Study the drawing (mm; zero at the part's minimum x, y, z) and answer. A direction names the side the tool comes from. Give positions to 0.01 mm unless a question says otherwise; leave off trailing zeros. Loops run counter-clockwise (first coordinate to the right, second up) from the corner with the lowest first, then second, coordinate; pieces in that order, holes last. Notation, with made-up numbers: (70.25, 45.25) - (78.25, 45.25) arc R12 cw to (78.25, 61.25) - close; hole circle Ø1 at (58, -36.75). An arc over 180 degrees is marked (long way). One line per item, written item: value. Start each with the question number.
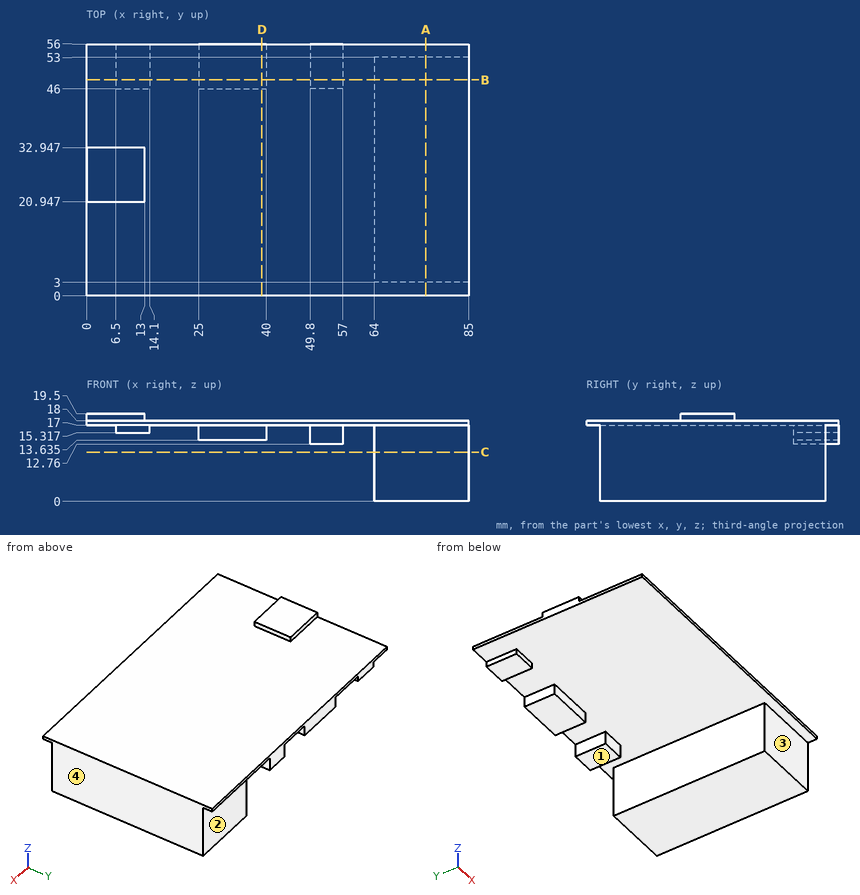
1. A cutting plane is placed at A-A (x = 75.5). Determine the outline of the cut face in (y, z), plus the area to 3 significant figures.
2. A cutting plane is placed at C-C (z = 11). Determine the outline of the cut face in (x, y), plus the area to 3 significant figures.
3. Find the intervals of material crossed by L1, parallel to Z at x = 63.5, y = 16.5; L2, parallel to X at y = 36, z = 3.75; L3, parallel to Z at x = 75, y = 51.5, in increasing order. Write a range as [from, to].
4. For the marked faces 1, 2, 3 and 4, determine the directions among +Z, -Z, +X, -X, +Y, -Y from which every point of the face is accessible in a straight line to the end or side of a thin tool.
5. Flat-ended cylindrical pins translate along their axes: pin 1 (3.5 mm diameter, centred on y = 53.5, z = 14, fed in from -X); pin 2 (1.3 mm diameter, centred on x = 12, z = 16, fed in from -Y); pin 3 (2 mm diameter, centred on x = 76, z = 6.5, fed in from +Y); pin 4 (3 mm diameter, centred on x = 23, z = 11, fed in from -Y). Find the tip coordinate at first contact, or state that the pin passes through.
6. A cutting plane is placed at D-D (x = 39). Determine the outline of the cut face in (y, z) (1 decimal).
7. A cutting plane is placed at B-B (y = 48). Determine the outline of the cut face in (x, z) (1 decimal).
Results below:
1. outline: (0, 17) - (3, 17) - (3, 0) - (53, 0) - (53, 17) - (56, 17) - (56, 18) - (0, 18) - close
1. area: 906 mm^2
2. outline: (64, 3) - (85, 3) - (85, 53) - (64, 53) - close
2. area: 1,050 mm^2
3. L1: z = [17, 18]
3. L2: x = [64, 85]
3. L3: z = [0, 18]
4. face 1: -Z, -X, +Y, -Y
4. face 2: -Z, +X, +Y
4. face 3: -Z, +X, -X, -Y
4. face 4: +Z, -Z, +X, +Y, -Y
5. pin 1: stops at x = 6.5
5. pin 2: stops at y = 46
5. pin 3: stops at y = 53
5. pin 4: passes through
6. outline: (0, 17) - (46, 17) - (46, 13.6) - (56, 13.6) - (56, 18) - (0, 18) - close
7. outline: (0, 17) - (6.5, 17) - (6.5, 15.3) - (14.1, 15.3) - (14.1, 17) - (25, 17) - (25, 13.6) - (40, 13.6) - (40, 17) - (49.8, 17) - (49.8, 12.8) - (57, 12.8) - (57, 17) - (64, 17) - (64, 0) - (85, 0) - (85, 18) - (0, 18) - close
